from build123d import *
from build123d.topology import SkipClean

# Parameters (mm, degrees)
SKETCH1_W           = 22.8
SKETCH1_H           = 12
BOSS_EXTRUDE1_DEPTH = 3
SKETCH2_R           = 56.4
SKETCH2_R_2         = 40.6
SKETCH2_R_3         = 37
SKETCH2_W           = 22.8
SKETCH2_H           = 12
BOSS_EXTRUDE2_DEPTH = 6.5
FILLET1_R           = 8
SKETCH3_W           = 5.3
SKETCH3_H           = 12
SKETCH3_R           = 0.6
BOSS_EXTRUDE3_DEPTH = 6.1
CHAMFER1_SIZE       = 2
SKETCH4_W           = 12.561985035
SKETCH4_H           = 13.525375378
CUT_EXTRUDE1_DEPTH  = 1
SKETCH5_R           = 2
CUT_EXTRUDE2_DEPTH  = 4
CUT_EXTRUDE3_DEPTH  = 11.9
SKETCH7_R           = 7.5
CUT_EXTRUDE4_DEPTH  = 10
BOSS_EXTRUDE4_DEPTH = 12
BOSS_EXTRUDE5_DEPTH = 3
CUT_EXTRUDE5_DEPTH  = 12


with BuildPart() as part:
    # Sketch1 → Boss-Extrude1 (new body)
    with BuildSketch(Plane(origin=(0, 0, 0), x_dir=(1, 0, 0), z_dir=(0, 1, 0))):
        with BuildLine():
            Line((112, 55), (112, -55))
            Line((112, -55), (23.979157617, -55))
            ThreePointArc((23.979157617, -55), (-60, 0), (23.979157617, 55))
            Line((23.979157617, 55), (112, 55))
        make_face()
        with Locations((5.4, 0)):
            Rectangle(SKETCH1_W, SKETCH1_H, mode=Mode.SUBTRACT)
    extrude(amount=BOSS_EXTRUDE1_DEPTH)

    # Sketch2 → Boss-Extrude2 (add)
    # profile 1 of 4: a face of its own
    with SkipClean():  # the faces are left unmerged after this step: merging them gives an invalid solid
        with BuildSketch(Plane(origin=(0, 3, 0), x_dir=(1, 0, 0), z_dir=(0, 1, 0))):
            with BuildLine():
                ThreePointArc((23.979157617, -55), (50.193373352, -32.872865277), (60, 0))
                ThreePointArc((60, 0), (50.193373352, 32.872865277), (23.979157617, 55))
                ThreePointArc((23.979157617, 55), (-60, 0), (23.979157617, -55))
            make_face()
            with Locations(Location((0, 0, 0), (0, 0, 90))):
                Circle(SKETCH2_R, mode=Mode.SUBTRACT)
        # profile 2 of 4: a face of its own
        with BuildSketch(Plane(origin=(0, 3, 0), x_dir=(1, 0, 0), z_dir=(0, 1, 0))):
            with Locations(Location((0, 0, 0), (0, 0, 90))):
                Circle(SKETCH2_R_2)
            with Locations(Location((0, 0, 0), (0, 0, 90))):
                Circle(SKETCH2_R_3, mode=Mode.SUBTRACT)
        # profile 3 of 4: a face of its own
        with BuildSketch(Plane(origin=(0, 3, 0), x_dir=(1, 0, 0), z_dir=(0, 1, 0))):
            with Locations((5.4, 0)):
                Rectangle(SKETCH2_W, SKETCH2_H)
        # profile 4 of 4: a face of its own
        with BuildSketch(Plane(origin=(0, 3, 0), x_dir=(1, 0, 0), z_dir=(0, 1, 0))):
            with Locations((5.4, 0)):
                Rectangle(SKETCH2_W, SKETCH2_H)
        extrude(amount=BOSS_EXTRUDE2_DEPTH)


with BuildPart() as boss_extrude2_kept_piece:
    # of the separate pieces the step leaves, the one the design keeps (boss_extrude2_pieces_kept)
    add(part.part.solids().sort_by_distance((23.979157617, 0, -55))[0])

    # Fillet1
    # the kernel refuses this fillet: 8 mm, written as the material it adds along each edge
    with BuildSketch(Plane(origin=(0, 3, 0), x_dir=(0, 0, -1), z_dir=(1, 0, 0))) as fillet1_piece_1:
        with BuildLine():
            CenterArc((48.541883177, 8), FILLET1_R, 270, 79.193077125)
            Line((48.541883177, 0), (48.541883177, -0.16))
            Line((48.541883177, -0.16), (56.4, -0.16))
            Line((56.4, -0.16), (56.56, 0))
            ThreePointArc((56.56, 0), (56.56, 3.25), (56.557162336, 6.47))
            Line((56.557162336, 6.47), (56.4, 6.5))
        make_face()
    revolve(axis=Axis((0, 3, 0), (0, 1, 0)))
    with BuildSketch(Plane(origin=(0, 3, 0), x_dir=(0, 0, -1), z_dir=(1, 0, 0))) as fillet1_piece_2:
        with BuildLine():
            CenterArc((48.458116823, 8), FILLET1_R, 190.806922875, 79.193077125)
            Line((40.6, 6.5), (40.442837664, 6.47))
            ThreePointArc((40.442837664, 6.47), (40.44, 3.25), (40.44, 0))
            Line((40.44, 0), (40.6, -0.16))
            Line((40.6, -0.16), (48.458116823, -0.16))
            Line((48.458116823, -0.16), (48.458116823, 0))
        make_face()
    revolve(axis=Axis((0, 3, 0), (0, 1, 0)))

    # Sketch3 → Boss-Extrude3 (add)
    # profile 1 of 2: a face of its own
    with BuildSketch(Plane(origin=(0, 3, 0), x_dir=(1, 0, 0), z_dir=(0, 1, 0))):
        with Locations((-8.65, 0)):
            Rectangle(SKETCH3_W, SKETCH3_H)
        with Locations(Location((-8.35, 0, 0), (0, 0, 270))):
            Circle(SKETCH3_R, mode=Mode.SUBTRACT)
    # profile 2 of 2: a face of its own
    with BuildSketch(Plane(origin=(0, 3, 0), x_dir=(1, 0, 0), z_dir=(0, 1, 0))):
        with Locations((19.45, 0)):
            Rectangle(SKETCH3_W, SKETCH3_H)
        with Locations(Location((19.156, 0, 0), (0, 0, 270))):
            Circle(SKETCH3_R, mode=Mode.SUBTRACT)
    extrude(amount=BOSS_EXTRUDE3_DEPTH)

    # Chamfer1
    chamfer1_edges = [boss_extrude2_kept_piece.edges().sort_by_distance(p)[0] for p in [
        (112, 0, 0),
        (67.989578808, 0, 55),
        (-60, 0, 0),
        (67.989578808, 0, -55),
    ]]
    chamfer(chamfer1_edges, length=CHAMFER1_SIZE)

    # Sketch4 → Cut-Extrude1 (cut)
    with SkipClean():  # the faces are left unmerged after this step: merging them gives an invalid solid
        with BuildSketch(Plane.XZ):
            with Locations((68.298400031, 49.537890064)):
                Rectangle(SKETCH4_W, SKETCH4_H)
        extrude(amount=-CUT_EXTRUDE1_DEPTH, mode=Mode.SUBTRACT)

    # Sketch5 → Cut-Extrude2 (cut)
    with SkipClean():  # the faces are left unmerged after this step: merging them gives an invalid solid
        with BuildSketch(Plane.XZ):
            with Locations(Location((-39.5, 0, 0), (0, 0, 270))):
                Circle(SKETCH5_R)
            with Locations(Location((19.75, 34.208003449, 0), (0, 0, 270))):
                Circle(SKETCH5_R)
            with Locations(Location((19.75, -34.208003449, 0), (0, 0, 270))):
                Circle(SKETCH5_R)
        extrude(amount=-CUT_EXTRUDE2_DEPTH, mode=Mode.SUBTRACT)

    # Sketch6 → Cut-Extrude3 (cut)
    with SkipClean():  # the faces are left unmerged after this step: merging them gives an invalid solid
        with BuildSketch(Plane(origin=(0, 3, 0), x_dir=(1, 0, 0), z_dir=(0, 1, 0))):
            with BuildLine():
                Line((-28.714918284, 12), (0, 12))
                Line((0, 12), (28.714918284, 12))
                ThreePointArc((28.714918284, 12), (0, 31.121480236), (-28.714918284, 12))
            make_face()
            with BuildLine():
                Line((28.714918284, -12), (-28.714918284, -12))
                ThreePointArc((-28.714918284, -12), (0, -31.121480236), (28.714918284, -12))
            make_face()
        extrude(amount=-CUT_EXTRUDE3_DEPTH, mode=Mode.SUBTRACT)

    # Sketch7 → Cut-Extrude4 (cut)
    with SkipClean():  # the faces are left unmerged after this step: merging them gives an invalid solid
        with BuildSketch(Plane(origin=(0, 3, 0), x_dir=(1, 0, 0), z_dir=(0, 1, 0))):
            with Locations(Location((76.511791502, 37.774024263, 0), (0, 0, 270))):
                Circle(SKETCH7_R)
        extrude(amount=-CUT_EXTRUDE4_DEPTH, mode=Mode.SUBTRACT)

    # Sketch7<3> → Boss-Extrude4 (add)
    with SkipClean():  # the faces are left unmerged after this step: merging them gives an invalid solid
        with BuildSketch(Plane(origin=(0, 3, 0), x_dir=(1, 0, 0), z_dir=(0, 1, 0))):
            with BuildLine():
                Line((66.511791502, 37.774024263), (69.011791502, 37.774024263))
                ThreePointArc((69.011791502, 37.774024263), (76.511791502, 45.274024263), (84.011791502, 37.774024263))
                Line((84.011791502, 37.774024263), (86.511791502, 37.774024263))
                ThreePointArc((86.511791502, 37.774024263), (76.511791502, 47.774024263), (66.511791502, 37.774024263))
            make_face()
        extrude(amount=BOSS_EXTRUDE4_DEPTH)

    # Sketch8 → Boss-Extrude5 (add)
    with SkipClean():  # the faces are left unmerged after this step: merging them gives an invalid solid
        with BuildSketch(Plane(origin=(0, 15, 0), x_dir=(1, 0, 0), z_dir=(0, 1, 0))):
            with BuildLine():
                Line((64.511791502, 37.774024263), (66.511791502, 37.774024263))
                ThreePointArc((66.511791502, 37.774024263), (76.511791502, 47.774024263), (86.511791502, 37.774024263))
                Line((86.511791502, 37.774024263), (88.511791502, 37.774024263))
                ThreePointArc((88.511791502, 37.774024263), (76.511791502, 49.774024263), (64.511791502, 37.774024263))
            make_face()
        extrude(amount=-BOSS_EXTRUDE5_DEPTH)

    # Sketch9 → Cut-Extrude5 (cut)
    with SkipClean():  # the faces are left unmerged after this step: merging them gives an invalid solid
        with BuildSketch(Plane(origin=(0, 3, 0), x_dir=(1, 0, 0), z_dir=(0, 1, 0))):
            with BuildLine():
                Line((34.719854758, -55), (46.340443844, -55))
                Line((46.340443844, -55), (46.340443844, -47.3))
                Line((46.340443844, -47.3), (37.77394627, -47.3))
                ThreePointArc((37.77394627, -47.3), (36.264905061, -48.466665635), (34.719854758, -49.585206487))
                Line((34.719854758, -49.585206487), (34.719854758, -55))
            make_face()
        extrude(amount=-CUT_EXTRUDE5_DEPTH, mode=Mode.SUBTRACT)


solid = boss_extrude2_kept_piece.part
Work out the finished part from the listing and answer in its coordinate system (mm). A direction names the side the tool comes from. Give positions to 0.01 mm unless a question says otherwise; leave off trailing zeros. Use a Markdown table: item, result. Add a question column.
1. Determine the mould class of faces 1 (the flat face through (78, 3, -1)), 2 (the flat face through (20, 4, -34)), 3 (the flat face through (86, 10, -37.774)) for opening direction Z: released by +Z, released by -Z, zero draft, split by the parting line, or undercut.
2. Section A-A on y = 6 is taken. State how many separate pieces and enclosed holes the cut face has, and give its area (3 significant figures).
3. Flat-ended cylindrical pins translate along their axes: pin 1 Ø0.9 at (x, y) = (-6.5, 1.5) entering from +Z; pin 2 Ø4.5 at (x, z) = (19.75, 34.21) entering from +Y; pin 3 Ø6 at (x, z) = (19.5, 1.5) entering from +Y. Find the tip coordinate at first contact, or state that the pin passes through.
4. For faces 4 (the flat face through (-9, 6, -6)), 5 (the flat face through (76, 15, -47)), 6 (the flat face through (-6, 4, 0)), 7 (the flat face through (-39, 4, 0)), 8 (the flat face through (76, 12, -48)), determine the directions among +Z, -Z, +X, -X, +Y, -Y from which every point of the face is accessible in a straight line to the end or side of a thin tool.
5. Find the intervals of material crossed by probe 1 along Z at (x, y) = (10, 6.5); probe 2 along X at (y, z) = (1.25, 0.5); probe 3 along X at (y, z) = (7, -8.5), in increasing order.
Results below:
| question | item | result |
|---|---|---|
| 1 | face 1 | zero draft |
| 1 | face 2 | undercut |
| 1 | face 3 | released by +Z |
| 2 | separate pieces | 5 |
| 2 | enclosed holes | 4 |
| 2 | area | 3,370 mm^2 |
| 3 | pin 1 | stops at z = 59.6 |
| 3 | pin 2 | stops at y = 9.5 |
| 3 | pin 3 | stops at y = 9.1 |
| 4 | face 4 | +Y |
| 4 | face 5 | +Z, -Z, +X, -X, +Y |
| 4 | face 6 | +Y, -Y |
| 4 | face 7 | -Y |
| 4 | face 8 | -Z |
| 5 | probe 1 | z = -59.16 to -54.24, -40.63 to -35.62, 35.62 to 40.63, 54.24 to 59.16 |
| 5 | probe 2 | x = -59.25 to -41.44, -37.56 to -6, 16.8 to 111.25 |
| 5 | probe 3 | x = -59.39 to -54.81, -40.65 to -36.01, 36.01 to 40.65, 54.81 to 59.39 |
